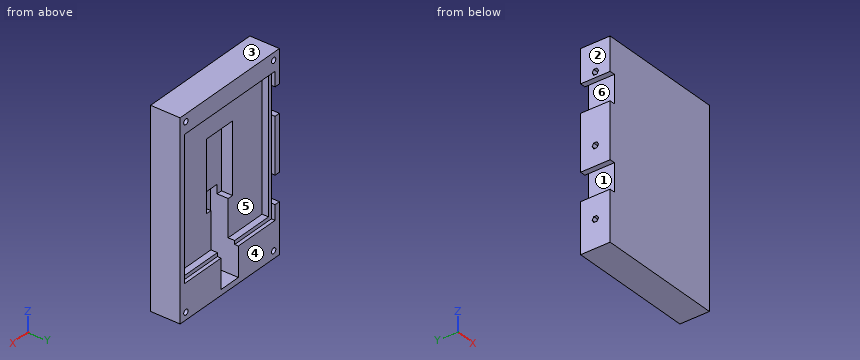
from build123d import *

# Parameters (mm, degrees)
SKETCH1_W           = 69
SKETCH1_H           = 105
BOSS_EXTRUDE1_DEPTH = 16
SKETCH2_W           = 63
SKETCH2_H           = 76
CUT_EXTRUDE1_DEPTH  = 2
SKETCH3_W           = 59
SKETCH3_H           = 72
CUT_EXTRUDE2_DEPTH  = 3.5
SKETCH4_W           = 18
SKETCH4_H           = 38
CUT_EXTRUDE3_DEPTH  = 6
SKETCH5_W           = 12
SKETCH5_H           = 31.473581166
CUT_EXTRUDE4_DEPTH  = 9.5
SKETCH6_W           = 12
SKETCH6_H           = 18
CUT_EXTRUDE5_DEPTH  = 15
SKETCH7_R           = 1.5
CUT_EXTRUDE6_DEPTH  = 10
CUT_EXTRUDE7_DEPTH  = 10
SKETCH13_W          = 3
SKETCH13_H          = 15
CUT_EXTRUDE8_DEPTH  = 17


with BuildPart() as part:
    # Sketch1 → Boss-Extrude1 (new body)
    with BuildSketch(Plane(origin=(0, 0, 0), x_dir=(1, 0, 0), z_dir=(0, 1, 0))):
        with Locations((34.5, 52.5)):
            Rectangle(SKETCH1_W, SKETCH1_H)
    extrude(amount=BOSS_EXTRUDE1_DEPTH)

    # Sketch2 → Cut-Extrude1 (cut)
    with BuildSketch(Plane(origin=(0, 16, 0), x_dir=(1, 0, 0), z_dir=(0, 1, 0))):
        with Locations((34.5, 48)):
            Rectangle(SKETCH2_W, SKETCH2_H)
    extrude(amount=-CUT_EXTRUDE1_DEPTH, mode=Mode.SUBTRACT)

    # Sketch3 → Cut-Extrude2 (cut)
    with BuildSketch(Plane(origin=(0, 14, 0), x_dir=(1, 0, 0), z_dir=(0, 1, 0))):
        with Locations((34.5, 48)):
            Rectangle(SKETCH3_W, SKETCH3_H)
    extrude(amount=-CUT_EXTRUDE2_DEPTH, mode=Mode.SUBTRACT)

    # Sketch4 → Cut-Extrude3 (cut)
    with BuildSketch(Plane(origin=(0, 10.5, 0), x_dir=(1, 0, 0), z_dir=(0, 1, 0))):
        with Locations((34.54, 45)):
            Rectangle(SKETCH4_W, SKETCH4_H)
    extrude(amount=-CUT_EXTRUDE3_DEPTH, mode=Mode.SUBTRACT)

    # Sketch5 → Cut-Extrude4 (cut)
    with BuildSketch(Plane(origin=(0, 10.5, 0), x_dir=(1, 0, 0), z_dir=(0, 1, 0))):
        with Locations((34.54, 74.837937429)):
            Rectangle(SKETCH5_W, SKETCH5_H)
    extrude(amount=-CUT_EXTRUDE4_DEPTH, mode=Mode.SUBTRACT)

    # Sketch6 → Cut-Extrude5 (cut)
    with BuildSketch(Plane(origin=(0, 16, 0), x_dir=(1, 0, 0), z_dir=(0, 1, 0))):
        with Locations((34.54, 93)):
            Rectangle(SKETCH6_W, SKETCH6_H)
    extrude(amount=-CUT_EXTRUDE5_DEPTH, mode=Mode.SUBTRACT)

    # Sketch7 → Cut-Extrude6 (cut)
    with BuildSketch(Plane(origin=(0, 16, 0), x_dir=(1, 0, 0), z_dir=(0, 1, 0))):
        with Locations((4, 4)):
            Circle(SKETCH7_R)
        with Locations((65, 4)):
            Circle(SKETCH7_R)
        with Locations((65, 101)):
            Circle(SKETCH7_R)
        with Locations((4, 101)):
            Circle(SKETCH7_R)
    extrude(amount=-CUT_EXTRUDE6_DEPTH, mode=Mode.SUBTRACT)

    # Sketch10 → Cut-Extrude7 (cut)
    with BuildSketch(Plane.ZY):
        Polygon((-90, 9.732050808), (-91.5, 8.866025404), (-91.5, 7.133974596), (-90, 6.267949192), (-88.5, 7.133974596), (-88.5, 8.866025404), align=None)
        Polygon((-52.5, 9.732050808), (-54, 8.866025404), (-54, 7.133974596), (-52.5, 6.267949192), (-51, 7.133974596), (-51, 8.866025404), align=None)
        Polygon((-15, 9.732050808), (-16.5, 8.866025404), (-16.5, 7.133974596), (-15, 6.267949192), (-13.5, 7.133974596), (-13.5, 8.866025404), align=None)
    extrude(amount=-CUT_EXTRUDE7_DEPTH, mode=Mode.SUBTRACT)

    # Sketch13 → Cut-Extrude8 (cut, through all)
    with BuildSketch(Plane(origin=(0, 16, 0), x_dir=(1, 0, 0), z_dir=(0, 1, 0))):
        with Locations((1.5, 70.5)):
            Rectangle(SKETCH13_W, SKETCH13_H)
        with Locations((1.5, 25.5)):
            Rectangle(SKETCH13_W, SKETCH13_H)
    extrude(amount=-CUT_EXTRUDE8_DEPTH, mode=Mode.SUBTRACT)


solid = part.part
Could you check a few things on this model? Use its own coordinates, in mm. Face numbers are marked on the shaded views. A direction names the side the tool comes from. Coordinates: 2 decimals unless noted, no trailing zeros. Order: outer loops, then holes, each group sorted by start corner. A loop starts at its lowest first (then second) coordinate and runs counter-clockwise, first axis right, second up. Notation, with made-up numbers: (-5.75, 88.25) - (40.25, 88.25) arc R20 ccw to (40.25, 122.25) - close; hole circle Ø9 at (52, -37). An arc over 180 degrees is marked (long way). Answer in a Markdown table with one row per item. Add a question column.
(1) On a 3-axis mill with a long thin cutter (end or side, diameter ignored), from which of +Z, -Z, +X, -X, +Y, -Y can I reach the whole of each face in a straight line? I mean the marked faces 4, 5 and 6. Say none if no direction works.
(2) I need wall thicknesses on L1, parallel to X at y = 13, z = -101; L2, parallel to Z at x = 65, y = 13.5; L3, parallel to Z at x = 4, y = 8. Which ranges of each line are inside material? Lowest first, please.
(3) If we section it at D-D, the plane x = 27.5: Please give me the cut outline in (y, z), then the cut area to 3 significant figures.
(4) Will these pins go through, and if not, where does the flat tip stop? pin 1 (3.5 mm diameter, centred on x = 1.5, y = 11, fed in from +Z); pin 2 (1.5 mm diameter, centred on x = 65.5, z = -4.5, fed in from +Y); pin 3 (7 mm diameter, centred on y = 9.5, z = -24, fed in from -X); pin 4 (1.5 mm diameter, centred on x = 37.5, z = -68, fed in from +Y).
(5) If we section it at B-B, the plane y = 11.75: Please give me the cut outline in (x, z), then the cut area to 3 significant figures.
(6) If we section it at C-C, the plane z = -4: Please give me the cut outline in (x, y).
(7) If we section it at A-A, the plane x = 48.5: Please give me the cut outline in (y, z), then the cut area to 3 significant figures.
(8) If we mould it in two halves opening along Z, with no side actions, what happens to the marked faces 1, 2 and 3? For each: released by +Z, released by -Z, zero draft, split by the parting line, or undercut.
Results are:
| question | item | result |
|---|---|---|
| 1 | face 4 | +Z, -Z, +X, -X, +Y |
| 1 | face 5 | +Y |
| 1 | face 6 | -X, +Y, -Y |
| 2 | L1 | x = 0 to 2.5, 5.5 to 28.54, 40.54 to 63.5, 66.5 to 69 |
| 2 | L2 | z = -105 to -102.5, -99.5 to -5.5, -2.5 to 0 |
| 2 | L3 | z = -105 to -102.5, -99.5 to -91.5, -88.5 to -54, -51 to -16.5, -13.5 to -5.5, -2.5 to 0 |
| 3 | outline | (0, -105) - (16, -105) - (16, -86) - (14, -86) - (14, -84) - (10.5, -84) - (10.5, -64) - (4.5, -64) - (4.5, -26) - (10.5, -26) - (10.5, -12) - (14, -12) - (14, -10) - (16, -10) - (16, 0) - (0, 0) - close |
| 3 | area | 1,050 mm2 |
| 4 | pin 1 | stops at z = 0 |
| 4 | pin 2 | stops at y = 6 |
| 4 | pin 3 | stops at x = 3 |
| 4 | pin 4 | stops at y = 1 |
| 5 | outline | (0, -105) - (69, -105) - (69, 0) - (0, 0) - (0, -18) - (3, -18) - (3, -33) - (0, -33) - (0, -63) - (3, -63) - (3, -78) - (0, -78) - close; hole circle Ø3 at (4, -101); hole circle Ø3 at (4, -4); hole (5, -84) - (28.54, -84) - (28.54, -102) - (40.54, -102) - (40.54, -84) - (64, -84) - (64, -12) - (5, -12) - close; hole circle Ø3 at (65, -101); hole circle Ø3 at (65, -4) |
| 5 | area | 2,660 mm2 |
| 6 | outline | (0, 0) - (69, 0) - (69, 16) - (66.5, 16) - (66.5, 6) - (63.5, 6) - (63.5, 16) - (5.5, 16) - (5.5, 6) - (2.5, 6) - (2.5, 16) - (0, 16) - close |
| 7 | outline | (0, -105) - (16, -105) - (16, -86) - (14, -86) - (14, -84) - (10.5, -84) - (10.5, -12) - (14, -12) - (14, -10) - (16, -10) - (16, 0) - (0, 0) - close |
| 7 | area | 1,280 mm2 |
| 8 | face 1 | undercut |
| 8 | face 2 | zero draft |
| 8 | face 3 | released by +Z |
